Check sheet for the drawn part. Datum: minimum x, y, z corner. Units: mm. Coordinates: 2 decimals unless noted, no trailing zeros. Write each loop counter-clockwise with the first axis right and the second up, starting at its lowest first coordinate (ties: lowest second). Pieces come first, ordered by that corner, then holes. Notation, with made-up numbers: M -1,28 L 58,28 A29 ccw 58,63 Z; hole C -33,67 d10. An arc over 180 degrees is marked long. Answer as CSV lines item,"result". Start each with the question number.
Q1. Sectioned sample at D-D, the plane y = 11.5. Record the cut outline in (x, z), then the cut area to 3 significant figures.
Q2. Sectioned sample at A-A, the plane x = 36. Record the cut outline in (y, z).
Q3. Sectioned sample at B-B, the plane z = 3.5. Record the cut outline in (x, y).
Q4. Sectioned sample at C-C, the plane y = 68. Record the cut outline in (x, z), then the cut area to 3 significant figures.
Q5. Thickness scan on line 1 along X through (y, z) = (38, 3.25); line 2 along Y through (x, z) = (61, 0.5); line 3 along X through (y, z) = (9, 5.5). Record the ranges inside material, lowest first. Write a range as from..to.
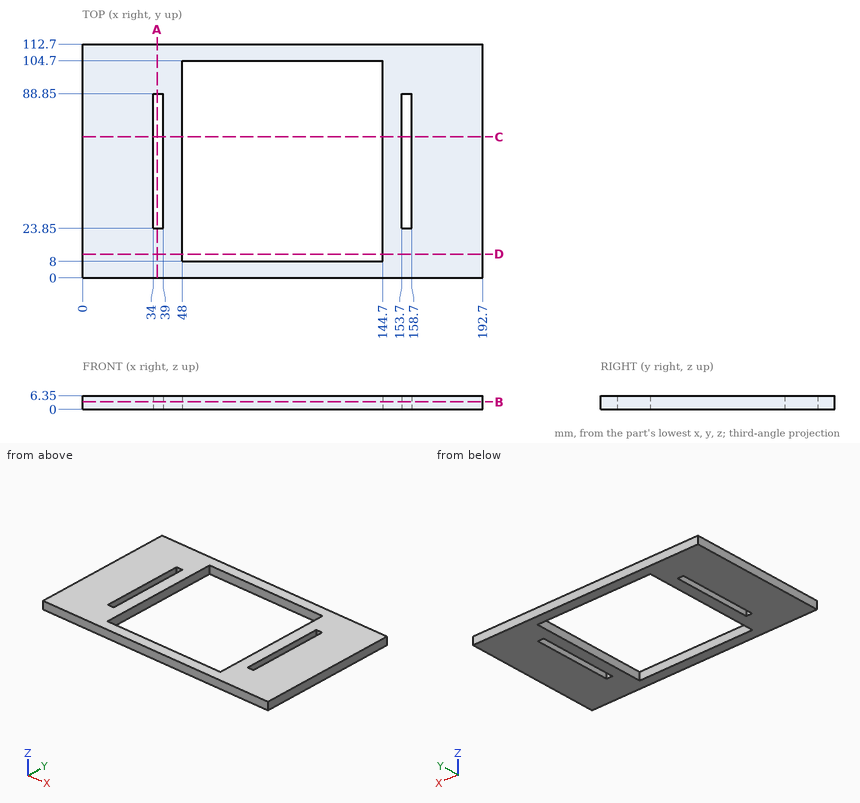
Output:
1,outline,"M 0,0 L 48,0 L 48,6.35 L 0,6.35 Z; M 144.7,0 L 192.7,0 L 192.7,6.35 L 144.7,6.35 Z"
1,area,"610 mm^2"
2,outline,"M 0,0 L 23.85,0 L 23.85,6.35 L 0,6.35 Z; M 88.85,0 L 112.7,0 L 112.7,6.35 L 88.85,6.35 Z"
3,outline,"M 0,0 L 192.7,0 L 192.7,112.7 L 0,112.7 Z; hole M 34,23.85 L 39,23.85 L 39,88.85 L 34,88.85 Z; hole M 48,8 L 144.7,8 L 144.7,104.7 L 48,104.7 Z; hole M 153.7,23.85 L 158.7,23.85 L 158.7,88.85 L 153.7,88.85 Z"
4,outline,"M 0,0 L 34,0 L 34,6.35 L 0,6.35 Z; M 39,0 L 48,0 L 48,6.35 L 39,6.35 Z; M 144.7,0 L 153.7,0 L 153.7,6.35 L 144.7,6.35 Z; M 158.7,0 L 192.7,0 L 192.7,6.35 L 158.7,6.35 Z"
4,area,"546 mm^2"
5,line 1,"x = 0..34, 39..48, 144.7..153.7, 158.7..192.7"
5,line 2,"y = 0..8, 104.7..112.7"
5,line 3,"x = 0..48, 144.7..192.7"
